Part model, mm, in its own coordinate system. A direction names the side the tool comes from. Give positions to 0.01 mm unless a question says otherwise; leave off trailing zeros. Order: outer loops, then holes, each group sorted by start corner. A loop starts at its lowest first (then second) coordinate and runs counter-clockwise, first axis right, second up. Notation, with made-up numbers: M -37.75,42.5 L 17.25,42.5 A20 ccw 17.25,55.5 Z; hole C -17,29 d6. An arc over 180 degrees is marked long. Answer as a JSON object with one key per item and string values.
from build123d import *

# Parameters (mm, degrees)
SKETCH1_W           = 42.299999982
SKETCH1_H           = 42.299999982
BOSS_EXTRUDE1_DEPTH = 42.8625
SKETCH2_R           = 2
CUT_EXTRUDE1_DEPTH  = 6.35
CHAMFER1_SIZE       = 3.81
SKETCH3_R           = 2.5
BOSS_EXTRUDE2_DEPTH = 24


with BuildPart() as part:
    # Sketch1 → Boss-Extrude1 (new body)
    with BuildSketch(Plane(origin=(0, 0, 0), x_dir=(1, 0, 0), z_dir=(0, 1, 0))):
        Rectangle(SKETCH1_W, SKETCH1_H)
    extrude(amount=BOSS_EXTRUDE1_DEPTH)

    # Sketch2 → Cut-Extrude1 (cut)
    with BuildSketch(Plane(origin=(0, 42.8625, 0), x_dir=(1, 0, 0), z_dir=(0, 1, 0))):
        with Locations((-15.499999988, -15.499999988)):
            Circle(SKETCH2_R)
        with Locations((-15.499999988, 15.499999988)):
            Circle(SKETCH2_R)
        with Locations((15.499999988, 15.499999988)):
            Circle(SKETCH2_R)
        with Locations((15.499999988, -15.499999988)):
            Circle(SKETCH2_R)
    extrude(amount=-CUT_EXTRUDE1_DEPTH, mode=Mode.SUBTRACT)

    # Chamfer1
    chamfer1_edges = [part.edges().sort_by_distance(p)[0] for p in [
        (-21.149999991, 21.43125, -21.149999991),
        (21.149999991, 21.43125, -21.149999991),
        (21.149999991, 21.43125, 21.149999991),
        (-21.149999991, 21.43125, 21.149999991),
    ]]
    chamfer(chamfer1_edges, length=CHAMFER1_SIZE)

    # Sketch3 → Boss-Extrude2 (add)
    with BuildSketch(Plane(origin=(0, 42.8625, 0), x_dir=(1, 0, 0), z_dir=(0, 1, 0))):
        Circle(SKETCH3_R)
    extrude(amount=BOSS_EXTRUDE2_DEPTH)


solid = part.part
1. Cut at B-B on y = 34.5. Give the cut face in (x, z).
Worked answers:
{"outline": "M -21.15,-17.34 L -17.34,-21.15 L 17.34,-21.15 L 21.15,-17.34 L 21.15,17.34 L 17.34,21.15 L -17.34,21.15 L -21.15,17.34 Z"}
2. Which spindle directions (+Z, -Z, +X, -X, +Y, -Y) get a long thin tool onto all of the face, cutting with end or side? Do faces 4 (the flat face through (0, 21, 21.15)), 5 (the flat face through (15, 36.512, -16)). Say none if no direction does.
Worked answers:
{"face 4": "+Z, +X, -X, +Y, -Y", "face 5": "+Y"}
3. Cut at C-C on z = -15.5. Give the cut face in (x, y).
Worked answers:
{"outline": "M -21.15,0 L 21.15,0 L 21.15,42.86 L 17.5,42.86 L 17.5,36.51 L 13.5,36.51 L 13.5,42.86 L -13.5,42.86 L -13.5,36.51 L -17.5,36.51 L -17.5,42.86 L -21.15,42.86 Z"}
4. Cut at A-A on x = -15.5. Give the cut face in (y, z).
Worked answers:
{"outline": "M 0,-21.15 L 42.86,-21.15 L 42.86,-17.5 L 36.51,-17.5 L 36.51,-13.5 L 42.86,-13.5 L 42.86,13.5 L 36.51,13.5 L 36.51,17.5 L 42.86,17.5 L 42.86,21.15 L 0,21.15 Z"}
5. Cut at D-D on x = 0. Give the cut face in (y, z), plus the area to 3 significant figures.
Worked answers:
{"outline": "M 0,-21.15 L 42.86,-21.15 L 42.86,-2.5 L 66.86,-2.5 L 66.86,2.5 L 42.86,2.5 L 42.86,21.15 L 0,21.15 Z", "area": "1,930 mm^2"}
6. Two-plate mould, pull along X, no slides. Class faces 1 (the flat face through (15, 36.512, 15)), 2 (the flat face through (19.27, 21.13, -19.22)), 3 (the flat face through (0, 21, -21.15)): +X half, -X half, draft (parallel to the pull), parting line (faces both ways), or undercut.
Worked answers:
{"face 1": "undercut", "face 2": "+X half", "face 3": "draft"}
7. Probe line 1 along X through (y, z) = (41.75, 15.5); line 2 along Y through (x, z) = (-8.5, 3). List the from-to ranges inside material, lowest first.
Worked answers:
{"line 1": "x = -21.15 to -17.5, -13.5 to 13.5, 17.5 to 21.15", "line 2": "y = 0 to 42.86"}
8. Pin check, flat tips, straight feed: P1, Ø4.5, axis at x = -16.5, z = -15.5, coming from the +Y side; P2, Ø2, axis at x = 15.5, z = 16, coming from the +Y side. Stop position of each tip, or through.
Worked answers:
{"P1": "stops at y = 42.86", "P2": "stops at y = 36.51"}
